Autodesk Inventor part; units mm, degrees
ref_plane "YZ Plane" through (0, 0, 0) normal (1, 0, 0) x (0, 1, 0)
ref_plane "XZ Plane" through (0, 0, 0) normal (0, 1, 0) x (-1, 0, 0)
ref_plane "XY Plane" through (0, 0, 0) normal (0, 0, 1) x (1, 0, 0)
sketch "Sketch7" plane through (0, 0, 0) normal (0, 0, 1) x (1, 0, 0)
  line L0 (0, 0) -> (-80, 0)
  line L1 (-80, 0) -> (-80, 80)
  line L2 (-80, 80) -> (0, 80)
  line L3 (0, 80) -> (0, 0)
  line L4 (-70, 10) -> (-10, 10)
  line L5 (-10, 10) -> (-10, 70)
  line L6 (-10, 70) -> (-70, 70)
  line L7 (-70, 70) -> (-70, 10)
  dimension "d54" = 80
  dimension "d55" = 80
  dimension "d110" = 60
  dimension "d111" = 60
extrude "Extrusion10" add sketch "Sketch7" along normal blind 60 contours L0 L1 L2 L3 | L7 L6 L5 L4
sketch "Sketch8" plane through (0, 0, 60) normal (0, 0, 1) x (1, 0, 0)
  line L0 (0, 0) -> (0, 80)
  line L1 (0, 0) -> (-80, 0)
  line L2 (-80, 0) -> (-80, 80)
  line L3 (-80, 80) -> (0, 80)
  line L4 (0, 80) -> (0, 0)
  dimension "d60" = 80
  dimension "d61" = 80
extrude "Extrusion11" add sketch "Sketch8" along normal blind 5
sketch "Sketch9" plane through (0, 0, 65) normal (0, 0, 1) x (1, 0, 0)
  line L0 (-12.5, 12.5) -> (-67.5, 12.5)
  line L1 (-67.5, 12.5) -> (-67.5, 67.5)
  line L2 (-67.5, 67.5) -> (-12.5, 67.5)
  line L3 (-12.5, 67.5) -> (-12.5, 12.5)
  point P0 (0, 0)
  dimension "d64" = 55
  dimension "d65" = 55
extrude "Extrusion12" cut sketch "Sketch9" against normal blind 2
sketch "Sketch10" plane through (0, 0, 0) normal (1, 0, 0) x (0, 0, -1)
  line L0 (-63.5, 12.5) -> (-8.5, 12.5)
  line L1 (-8.5, 12.5) -> (-8.5, 67.5)
  line L2 (-8.5, 67.5) -> (-63.5, 67.5)
  line L3 (-63.5, 67.5) -> (-63.5, 12.5)
  point P0 (0, 0)
  dimension "d68" = 55
  dimension "d69" = 55
extrude "Extrusion13" cut sketch "Sketch10" against normal blind 2
sketch "Sketch11" plane through (-80, 80, 0) normal (0, 1, 0) x (1, 0, 0)
  line L0 (12.5, -63.5) -> (67.5, -63.5)
  line L1 (67.5, -63.5) -> (67.5, -8.5)
  line L2 (67.5, -8.5) -> (12.5, -8.5)
  line L3 (12.5, -8.5) -> (12.5, -63.5)
  point P0 (80, 0)
  dimension "d72" = 55
  dimension "d73" = 55
sketch "Sketch12" plane through (-80, 0, 0) normal (-1, 0, 0) x (0, 0, 1)
  line L0 (63.5, 12.5) -> (8.5, 12.5)
  line L1 (8.5, 12.5) -> (8.5, 67.5)
  line L2 (8.5, 67.5) -> (63.5, 67.5)
  line L3 (63.5, 67.5) -> (63.5, 12.5)
  point P0 (0, 0)
  dimension "d74" = 55
  dimension "d75" = 55
sketch "Sketch13" plane through (-80, 0, 0) normal (0, -1, 0) x (1, 0, 0)
  line L0 (12.5, 63.5) -> (67.5, 63.5)
  line L1 (67.5, 63.5) -> (67.5, 8.5)
  line L2 (67.5, 8.5) -> (12.5, 8.5)
  line L3 (12.5, 8.5) -> (12.5, 63.5)
  point P0 (80, 0)
  dimension "d76" = 55
  dimension "d77" = 55
extrude "Extrusion14" cut sketch "Sketch11" against normal blind 2
extrude "Extrusion15" cut sketch "Sketch12" against normal blind 2
extrude "Extrusion16" cut sketch "Sketch13" against normal blind 2
sketch "Sketch14" plane through (-80, 80, 0) normal (0, 1, 0) x (1, 0, 0)
  line L0 (79, -1) -> (68.4, -1)
  line L1 (68.4, -1) -> (68.4, -6.6)
  line L2 (68.4, -6.6) -> (79, -6.6)
  line L3 (79, -6.6) -> (79, -1)
  line L4 (1, -1) -> (11.6, -1)
  line L5 (11.6, -1) -> (11.6, -6.6)
  line L6 (11.6, -6.6) -> (1, -6.6)
  line L7 (1, -6.6) -> (1, -1)
  point P0 (80, 0)
  dimension "d84" = 10.6
  dimension "d85" = 5.6
  dimension "d86" = 10.6
  dimension "d87" = 5.6
extrude "Extrusion17" cut sketch "Sketch14" against normal blind 5
sketch "Sketch16" plane through (-80, 0, 0) normal (0, -1, 0) x (1, 0, 0)
  line L0 (1, 1) -> (11.6, 1)
  line L1 (11.6, 1) -> (11.6, 6.6)
  line L2 (11.6, 6.6) -> (1, 6.6)
  line L3 (1, 6.6) -> (1, 1)
  line L4 (79, 1) -> (68.4, 1)
  line L5 (68.4, 1) -> (68.4, 6.6)
  line L6 (68.4, 6.6) -> (79, 6.6)
  line L7 (79, 6.6) -> (79, 1)
  point P0 (80, 0)
  dimension "d94" = 10.6
  dimension "d95" = 5.6
  dimension "d96" = 10.6
  dimension "d97" = 5.6
extrude "Extrusion19" cut sketch "Sketch16" against normal blind 5
sketch "Sketch18" plane through (0, 0, 0) normal (0, 0, -1) x (-1, 0, 0)
  line L0 (10, 10) -> (70, 10)
  line L1 (70, 10) -> (70, 70)
  line L2 (70, 70) -> (10, 70)
  line L3 (10, 70) -> (10, 10)
  point P0 (0, 0)
  dimension "d114" = 60
  dimension "d115" = 60
extrude "Extrusion21" cut sketch "Sketch18" against normal blind 60
properties part number "Joint_MarkerCube_V3"
Source: CAD feature listing. Evaluate the final solid. Frame: model axes, mm. A direction names the side the tool comes from. Coordinates: 2 decimals unless noted, no trailing zeros. Write each loop counter-clockwise with the first axis right and the second up, starting at its lowest first coordinate (ties: lowest second). Pieces come first, ordered by that corner, then holes. Notation, with made-up numbers: M 45,61 L 73,61 A18 cw 73,87 Z; hole C 78.25,-7 d8. An arc over 180 degrees is marked long. Answer as a JSON object with one key per item and string values.
1. Cut plane B-B on y = 40.5. Output: boundary loops of the cut face in (x, z).
Evaluation:
{"outline": "M -80,0 L -70,0 L -70,60 L -10,60 L -10,0 L 0,0 L 0,8.5 L -2,8.5 L -2,63.5 L 0,63.5 L 0,65 L -12.5,65 L -12.5,63 L -67.5,63 L -67.5,65 L -80,65 L -80,63.5 L -78,63.5 L -78,8.5 L -80,8.5 Z"}
2. Cut plane C-C on x = -33. Output: boundary loops of the cut face in (y, z), plus the area to 3 significant figures.
Evaluation:
{"outline": "M 0,0 L 10,0 L 10,60 L 70,60 L 70,0 L 80,0 L 80,8.5 L 78,8.5 L 78,63.5 L 80,63.5 L 80,65 L 67.5,65 L 67.5,63 L 12.5,63 L 12.5,65 L 0,65 L 0,63.5 L 2,63.5 L 2,8.5 L 0,8.5 Z", "area": "1,270 mm^2"}
3. Contact query for flat-ended pins moving along their axis: P1, Ø0.6, axis at x = -78.5, z = 35.5, coming from the -Y side; P2, Ø5, axis at x = -60, y = 21.5, coming from the -Z side; P3, Ø4, axis at x = -45.5, z = 33.5, coming from the +Y side; P4, Ø3, axis at y = 46, z = 22, coming from the +X side. Output: stop coordinate, or through.
Evaluation:
{"P1": "y = 0", "P2": "z = 60", "P3": "y = 78", "P4": "x = -2"}
4. Ray query, L1, parallel to Y at x = -63.5, z = 54; L2, parallel to X at y = 58, z = 44.5; L3, parallel to X at y = 15, z = 3. Return the intervals inside material, ascending.
Evaluation:
{"L1": "2 to 10, 70 to 78", "L2": "-78 to -70, -10 to -2", "L3": "-80 to -70, -10 to 0"}
5. Draft query along Z for faces 1 (the flat face through (-1, 40, 63.5)), 2 (the flat face through (-40, 40, 63)), 3 (the flat face through (-43, 0, 8)). Return one class per face: released by +Z, released by -Z, zero draft, split by the parting line, or undercut.
Evaluation:
{"face 1": "undercut", "face 2": "released by +Z", "face 3": "zero draft"}
6. Cut plane A-A on z = 19. Output: boundary loops of the cut face in (x, y).
Evaluation:
{"outline": "M -80,0 L -67.5,0 L -67.5,2 L -12.5,2 L -12.5,0 L 0,0 L 0,12.5 L -2,12.5 L -2,67.5 L 0,67.5 L 0,80 L -12.5,80 L -12.5,78 L -67.5,78 L -67.5,80 L -80,80 L -80,67.5 L -78,67.5 L -78,12.5 L -80,12.5 Z; hole M -70,10 L -10,10 L -10,70 L -70,70 Z"}
7. Access query for faces 4 (the flat face through (-40, 67.5, 64)), 5 (the flat face through (-40, 70, 30)), 6 (the flat face through (-1, 2, 4)). Directions: +Z, -Z, +X, -X, +Y, -Y. A direction counts if a zero-diameter tool reaches every point of the face in a straight line with its end or side. Return the directions, or none.
Evaluation:
{"face 4": "+Z", "face 5": "-Z", "face 6": "-Y"}
